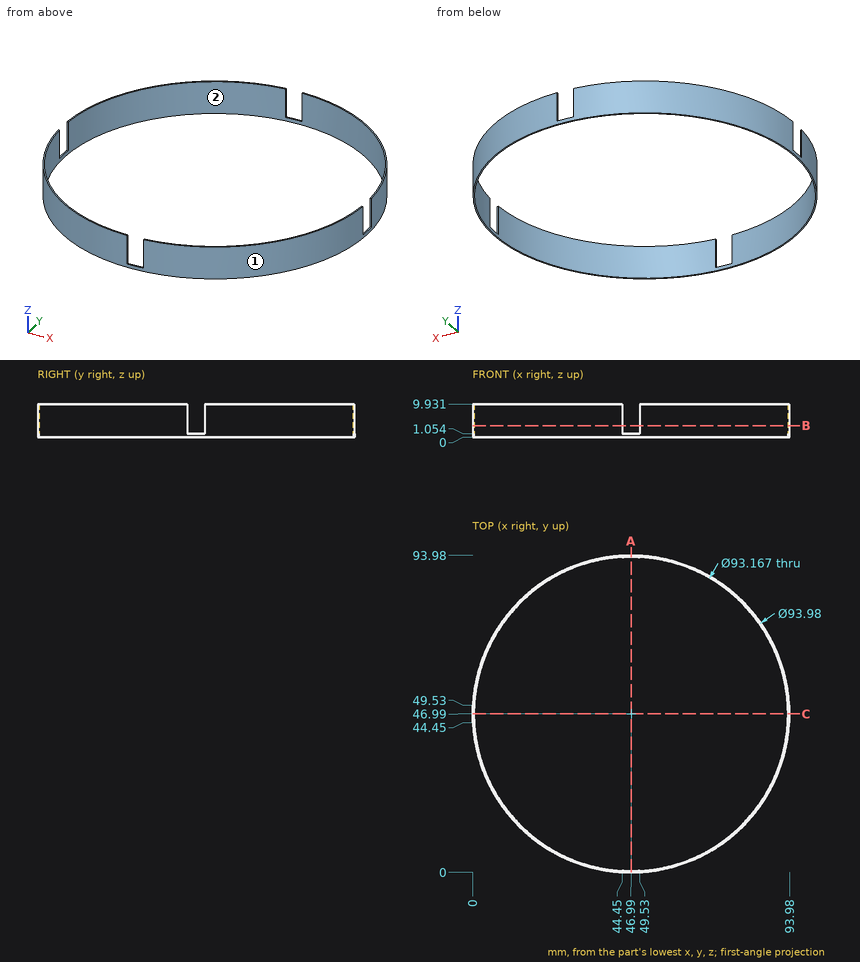
Geometry: see drawing. Coordinates: mm, zero at the bounding-box minimum. Coordinates: 2 decimals unless noted, no trailing zeros. Loops run counter-clockwise (first coordinate to the right, second up) from the corner with the lowest first, then second, coordinate; pieces in that order, holes last. Notation, with made-up numbers: (-4.75, -25.75) -> (49.25, -25.75) arc R10 ccw to (49.25, -13.75) -> close; hole circle Ø8 at (-7.75, -32). An arc over 180 degrees is marked (long way). Use a Markdown table: item, result.
1) Pull-direction query (X, two-part tool) for the marked faces 1 and 2; classes: released by +X, released by -X, zero draft, split by the parting line, or undercut.
Results found:
| item | result |
|---|---|
| face 1 | split by the parting line |
| face 2 | undercut |
2) Material intervals for line 1 along X through (y, z) = (45, 0.75); line 2 along Y through (x, z) = (44, 6.5) (1 decimal); line 3 along X through (y, z) = (53, 7.75) (1 decimal), sorted ascending. Write a range as from..to.
Results found:
| item | result |
|---|---|
| line 1 | x = 0.04..0.45, 93.53..93.94 |
| line 2 | y = 0.1..0.5, 93.5..93.9 |
| line 3 | x = 0.4..0.8, 93.2..93.6 |
3) Cut plane A-A (x = 46.99). Return the cut outline in (y, z).
Results found:
| item | result |
|---|---|
| outline | (0, 0) -> (0.41, 0) -> (0.41, 1.05) -> (0, 1.05) -> close; (93.57, 0) -> (93.98, 0) -> (93.98, 1.05) -> (93.57, 1.05) -> close |
4) Contact query for flat-ended pins moving along their axis: pin 1 (1.5 mm diameter, centred on y = 19, z = 4.5, fed in from -X); pin 2 (5 mm diameter, centred on x = 32.5, z = 8.5, fed in from -Y) (1 decimal); pin 3 (0.5 mm diameter, centred on x = 93.5, y = 47.5, fed in from +Z). Output: stop coordinate, or through.
Results found:
| item | result |
|---|---|
| pin 1 | stops at x = 8.7 |
| pin 2 | stops at y = 1.6 |
| pin 3 | stops at z = 1.05 |
5) Cut plane B-B (z = 3.5). Give the number of separate pieces and of enclosed holes in the cut face.
Results found:
| item | result |
|---|---|
| separate pieces | 4 |
| enclosed holes | 0 |
